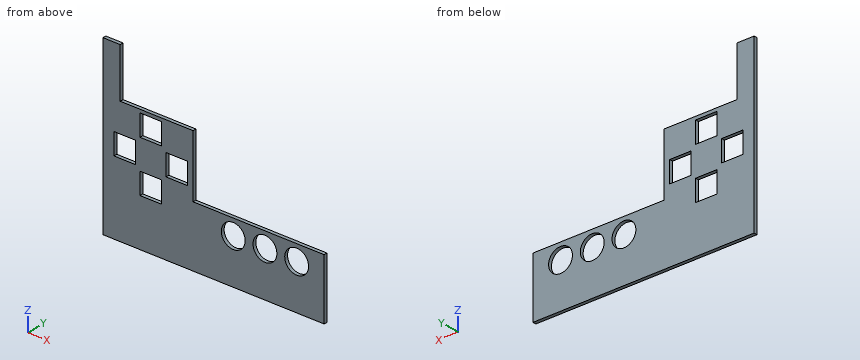
```python
from build123d import *

# Parameters (mm, degrees)
SKETCH1_W           = 64.85
SKETCH1_H           = 50.9
BOSS_EXTRUDE1_DEPTH = 1
SKETCH2_W           = 6.3
SKETCH2_H           = 6.3
SKETCH2_R           = 2.25
CUT_EXTRUDE1_DEPTH  = 10
SKETCH3_R           = 3.5
CUT_EXTRUDE2_DEPTH  = 10
CUT_EXTRUDE3_DEPTH  = 10


with BuildPart() as part:
    # Sketch1 → Boss-Extrude1 (new body)
    with BuildSketch(Plane(origin=(0, 0, 0), x_dir=(1, 0, 0), z_dir=(0, 1, 0))):
        Rectangle(SKETCH1_W, SKETCH1_H)
    extrude(amount=BOSS_EXTRUDE1_DEPTH)

    # Sketch2 → Cut-Extrude1 (cut)
    # profile 1 of 4: a face of its own
    with BuildSketch(Plane(origin=(0, 1, 0), x_dir=(1, 0, 0), z_dir=(0, 1, 0))):
        with Locations((-26.061755396, 0.805169379)):
            Rectangle(SKETCH2_W, SKETCH2_H)
        with Locations((-26.061755396, 0.805169379)):
            Circle(SKETCH2_R, mode=Mode.SUBTRACT)
    # profile 2 of 4: a face of its own
    with BuildSketch(Plane(origin=(0, 1, 0), x_dir=(1, 0, 0), z_dir=(0, 1, 0))):
        with Locations((-10.811755396, 0.805169379)):
            Rectangle(SKETCH2_W, SKETCH2_H)
        with Locations((-10.811755396, 0.805169379)):
            Circle(SKETCH2_R, mode=Mode.SUBTRACT)
    # profile 3 of 4: a face of its own
    with BuildSketch(Plane(origin=(0, 1, 0), x_dir=(1, 0, 0), z_dir=(0, 1, 0))):
        with Locations((-18.436755396, 8.330169379)):
            Rectangle(SKETCH2_W, SKETCH2_H)
        with Locations((-18.436755396, 8.330169379)):
            Circle(SKETCH2_R, mode=Mode.SUBTRACT)
    # profile 4 of 4: a face of its own
    with BuildSketch(Plane(origin=(0, 1, 0), x_dir=(1, 0, 0), z_dir=(0, 1, 0))):
        with Locations((-18.436755396, -6.719830621)):
            Rectangle(SKETCH2_W, SKETCH2_H)
        with Locations((-18.436755396, -6.719830621)):
            Circle(SKETCH2_R, mode=Mode.SUBTRACT)
    extrude(amount=-CUT_EXTRUDE1_DEPTH, mode=Mode.SUBTRACT)


with BuildPart() as cut_extrude1_kept_piece:
    # of the separate pieces the step leaves, the one the design keeps (cut_extrude1_pieces_kept)
    add(part.part.solids().sort_by_distance((32.425, 0, 25.45))[0])

    # Sketch3 → Cut-Extrude2 (cut)
    with BuildSketch(Plane(origin=(0, 1, 0), x_dir=(1, 0, 0), z_dir=(0, 1, 0))):
        with Locations(Location((5.766564163, 12.20008786, 0), (0, 0, 270))):
            Circle(SKETCH3_R)
        with Locations(Location((15.066564163, 12.20008786, 0), (0, 0, 270))):
            Circle(SKETCH3_R)
        with Locations(Location((24.366564163, 12.20008786, 0), (0, 0, 270))):
            Circle(SKETCH3_R)
    extrude(amount=-CUT_EXTRUDE2_DEPTH, mode=Mode.SUBTRACT)

    # Sketch6 → Cut-Extrude3 (cut)
    with BuildSketch(Plane(origin=(0, 1, 0), x_dir=(1, 0, 0), z_dir=(0, 1, 0))):
        Polygon((-6.013732281, -10.818181441), (-6.013732281, 7.549848679), (32.425, 7.549848679), (32.425, -25.45), (-27.388628542, -25.45), (-27.388628542, -10.818181441), align=None)
    extrude(amount=-CUT_EXTRUDE3_DEPTH, mode=Mode.SUBTRACT)


solid = cut_extrude1_kept_piece.part
```
The listing builds one solid part. Answer for the finished solid, in the listing's coordinates (mm). Round coordinates to 2 decimals unless told otherwise and drop trailing zeros. Loops run counter-clockwise (first coordinate to the right, second up) from the corner with the lowest first, then second, coordinate; pieces in that order, holes last. Notation, with made-up numbers: (75, 60) - (95, 60) arc R18 ccw to (95, 78) - close; hole circle Ø6 at (59.5, 33). An arc over 180 degrees is marked (long way). Return JSON: item names as keys, results as strings. Group by question number.
1. The part is cut by section A-A on z = 6. Determine the outline of the cut face in (x, y) (3 decimals).
2. Consider probe 1 along X at (y, z) = (0.15, 1.5) (3 decimals); probe 2 along X at (y, z) = (0.6, 5.5) (3 decimals); probe 3 along Z at (x, y) = (-25.5, 0.75). Determine where each line is inside the solid, lowest interval first.
3. The part is cut by section C-C on x = -18. Determine the outline of the cut face in (y, z), then the cut area to 3 significant figures.
4. Each of these flat-tipped pins is pushed along its axis until it touches: P1, Ø0.5, axis at x = -12.5, y = 0.5, coming from the +Z side; P2, Ø4, axis at x = 5.77, z = -12.2, coming from the +Y side. Where does it stop, or does it pass through?
5. The part is cut by section D-D on y = 0.15. Determine the outline of the cut face in (x, z) (3 decimals).
6. The part is cut by section B-B on x = -10. Determine the outline of the cut face in (y, z).
Resolved:
{
 "1": {"outline": "(-32.425, 0) - (-21.587, 0) - (-21.587, 1) - (-32.425, 1) - close; (-15.287, 0) - (-6.014, 0) - (-6.014, 1) - (-15.287, 1) - close"},
 "2": {"probe 1": "x = -32.425 to -29.212, -22.912 to -13.962, -7.662 to -6.014", "probe 2": "x = -32.425 to -21.587, -15.287 to -6.014", "probe 3": "z = -25.45 to -3.96, 2.34 to 10.82"},
 "3": {"outline": "(0, -25.45) - (1, -25.45) - (1, -11.48) - (0, -11.48) - close; (0, -5.18) - (1, -5.18) - (1, 3.57) - (0, 3.57) - close; (0, 9.87) - (1, 9.87) - (1, 10.82) - (0, 10.82) - close", "area": "23.7 mm²"},
 "4": {"P1": "stops at z = 10.82", "P2": "passes through"},
 "5": {"outline": "(-32.425, -25.45) - (32.425, -25.45) - (32.425, -7.55) - (-6.014, -7.55) - (-6.014, 10.818) - (-27.389, 10.818) - (-27.389, 25.45) - (-32.425, 25.45) - close; hole (-29.212, -3.955) - (-22.912, -3.955) - (-22.912, 2.345) - (-29.212, 2.345) - close; hole (-21.587, -11.48) - (-15.287, -11.48) - (-15.287, -5.18) - (-21.587, -5.18) - close; hole (-21.587, 3.57) - (-15.287, 3.57) - (-15.287, 9.87) - (-21.587, 9.87) - close; hole (-13.962, -3.955) - (-7.662, -3.955) - (-7.662, 2.345) - (-13.962, 2.345) - close; hole circle Ø7 at (5.767, -12.2); hole circle Ø7 at (15.067, -12.2); hole circle Ø7 at (24.367, -12.2)"},
 "6": {"outline": "(0, -25.45) - (1, -25.45) - (1, -3.96) - (0, -3.96) - close; (0, 2.34) - (1, 2.34) - (1, 10.82) - (0, 10.82) - close"}
}
